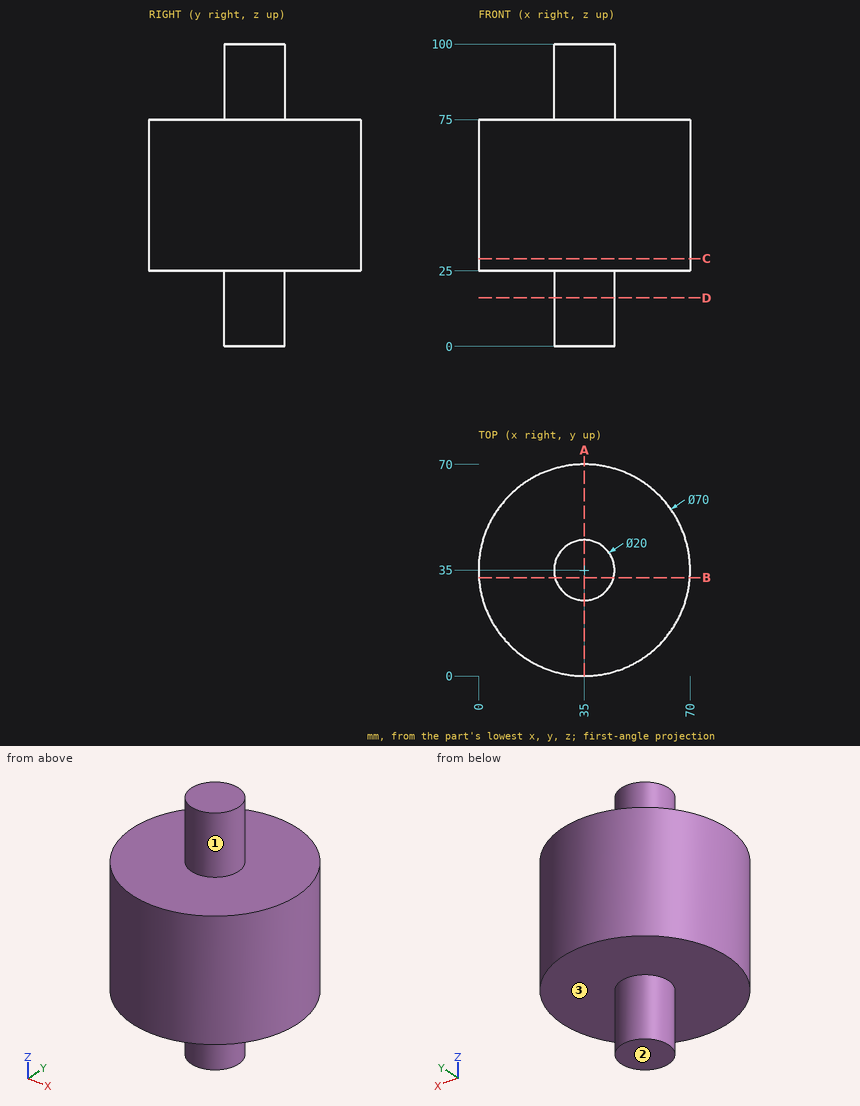
Input: dimensioned drawing with shaded views. Units: mm. Origin: part minimum x, y, z. A direction names the side the tool comes from. Coordinates: 2 decimals unless noted, no trailing zeros. Order: outer loops, then holes, each group sorted by start corner. A loop starts at its lowest first (then second) coordinate and runs counter-clockwise, first axis right, second up.
Item 1: Access query for the marked faces 1, 2 and 3. Directions: +Z, -Z, +X, -X, +Y, -Y. A direction counts if a zero-diameter tool reaches every point of the face in a straight line with its end or side. Return the directions, or none.
Answer:
face 1: +Z
face 2: -Z, +X, -X, +Y, -Y
face 3: -Z
Item 2: Section query A-A (x = 35). Output: boundary loops of the cut face in (y, z).
Answer:
outline: (0, 25) - (25, 25) - (25, 0) - (45, 0) - (45, 25) - (70, 25) - (70, 75) - (45, 75) - (45, 100) - (25, 100) - (25, 75) - (0, 75) - close
Item 3: Section query C-C (z = 29). Output: boundary loops of the cut face in (x, y).
Answer:
outline: circle Ø70 at (35, 35)
Item 4: Material intervals for line 1 along Z through (x, y) = (23, 16); line 2 along Y through (x, z) = (29.5, 76); line 3 along X through (y, z) = (45, 61), sorted ascending.
Answer:
line 1: z = 25 to 75
line 2: y = 26.65 to 43.35
line 3: x = 1.46 to 68.54
Item 5: Section query B-B (y = 32.5). Output: boundary loops of the cut face in (x, z), then the cut area to 3 significant figures.
Answer:
outline: (0.09, 25) - (25.32, 25) - (25.32, 0) - (44.68, 0) - (44.68, 25) - (69.91, 25) - (69.91, 75) - (44.68, 75) - (44.68, 100) - (25.32, 100) - (25.32, 75) - (0.09, 75) - close
area: 4,460 mm2
Item 6: Contact query for flat-ended pins moving along their axis: P1, Ø5, axis at y = 37.5, z = 69, coming from the -X side; P2, Ø6, axis at x = 55.5, y = 19, coming from the +Z side; P3, Ø2, axis at y = 31, z = 50, coming from the -X side; P4, Ø1, axis at y = 43, z = 21, coming from the +X side. Output: stop coordinate, or through.
Answer:
P1: stops at x = 0
P2: stops at z = 75
P3: stops at x = 0.13
P4: stops at x = 41.61
Item 7: Section query D-D (z = 16). Output: boundary loops of the cut face in (x, y).
Answer:
outline: circle Ø20 at (35, 35)
